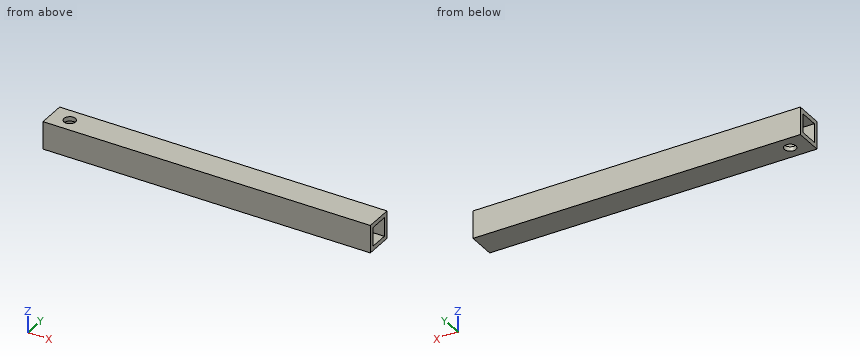
```python
from build123d import *

# Parameters (mm, degrees)
SKETCH1_W           = 19.05
SKETCH1_H           = 19.05
BOSS_EXTRUDE1_DEPTH = 112.7125
SHELL1_T            = -3.048
CUT_EXTRUDE2_REACH  = 116.707
SKETCH8_R           = 3.96875


with BuildPart() as part:
    # Sketch1 → Boss-Extrude1 (new, symmetric)
    with BuildSketch(Plane(origin=(0, 0, 0), x_dir=(0, 0, -1), z_dir=(1, 0, 0))):
        Rectangle(SKETCH1_W, SKETCH1_H)
    extrude(amount=BOSS_EXTRUDE1_DEPTH, both=True)

    # Shell1
    shell1_openings = [part.faces().sort_by_distance(p)[0] for p in [
        (112.7125, 0, 0),
        (-112.7125, 0, 0),
    ]]
    offset(amount=SHELL1_T, openings=shell1_openings, kind=Kind.INTERSECTION)

    # Cut-Extrude2: up to this face of the body (flat: up to its plane)
    cut_extrude2_end = Plane(part.part.faces().sort_by_distance((0, 0, 9.525))[0])
    # Sketch8 → Cut-Extrude2 (cut, up to the picked face)
    with BuildSketch(Plane(origin=(0, 0, -9.525), x_dir=(-1, 0, 0), z_dir=(0, 0, -1)), mode=Mode.PRIVATE) as cut_extrude2_sk1:
        with Locations(Location((100.0125, 0, 0), (0, 0, 90))):
            Circle(SKETCH8_R)
    cut_extrude2_tool1 = split(extrude(cut_extrude2_sk1.sketch, amount=-CUT_EXTRUDE2_REACH, mode=Mode.PRIVATE), bisect_by=cut_extrude2_end, keep=Keep.BOTH, mode=Mode.PRIVATE)
    add(cut_extrude2_tool1.solids().sort_by(Axis((-100.0125, 0, -9.525), (0, 0, 1)))[0], mode=Mode.SUBTRACT)


solid = part.part
```
The listing builds one solid part. Answer for the finished solid, in the listing's coordinates (mm). Coordinates: 2 decimals unless noted, no trailing zeros. Loops run counter-clockwise (first coordinate to the right, second up) from the corner with the lowest first, then second, coordinate; pieces in that order, holes last. Notation, with made-up numbers: (-5.5, 54) -> (10.5, 54) arc R31 ccw to (10.5, 87) -> close; hole circle Ø2 at (10.5, 20). An arc over 180 degrees is marked (long way). Return JSON: item names as keys, results as strings. Group by question number.
(1) A cutting plane is placed at A-A on x = 24. Write down the section's boundary in (y, z) (3 decimals).
(2) A cutting plane is placed at B-B on y = 0. Write down the section's boundary in (x, z) (1 decimal).
(3) A cutting plane is placed at C-C on z = -3.25. Write down the section's boundary in (x, y) (1 decimal).
(4) Find the intervals of material crossed by probe 1 along X at (y, z) = (0, -7.7); probe 2 along Z at (x, y) = (-8, 0.5) (3 decimals), in increasing order. Write a range as from..to.
The answers:
{
 "1": {"outline": "(-9.525, -9.525) -> (9.525, -9.525) -> (9.525, 9.525) -> (-9.525, 9.525) -> close; hole (-6.477, -6.477) -> (6.477, -6.477) -> (6.477, 6.477) -> (-6.477, 6.477) -> close"},
 "2": {"outline": "(-112.7, -9.5) -> (-104, -9.5) -> (-104, -6.5) -> (-112.7, -6.5) -> close; (-112.7, 6.5) -> (-104, 6.5) -> (-104, 9.5) -> (-112.7, 9.5) -> close; (-96, -9.5) -> (112.7, -9.5) -> (112.7, -6.5) -> (-96, -6.5) -> close; (-96, 6.5) -> (112.7, 6.5) -> (112.7, 9.5) -> (-96, 9.5) -> close"},
 "3": {"outline": "(-112.7, -9.5) -> (112.7, -9.5) -> (112.7, -6.5) -> (-112.7, -6.5) -> close; (-112.7, 6.5) -> (112.7, 6.5) -> (112.7, 9.5) -> (-112.7, 9.5) -> close"},
 "4": {"probe 1": "x = -112.71..-103.98, -96.04..112.71", "probe 2": "z = -9.525..-6.477, 6.477..9.525"}
}
